Here's the drawing with two shaded views (mm, measured from the low corner). I have some questions. Round coordinates to 2 decimals unless told otherwise and drop trailing zeros. Write each loop counter-clockwise with the first axis right and the second up, starting at its lowest first coordinate (ties: lowest second). Pieces come first, ordered by that corner, then holes. Notation, with made-up numbers: M 52,-0.75 L 95,-0.75 A27 cw 95,24.25 Z; hole C 81.25,54.5 d1. An arc over 180 degrees is marked long. Use one line per item in the form item = value. Start each with the question number.
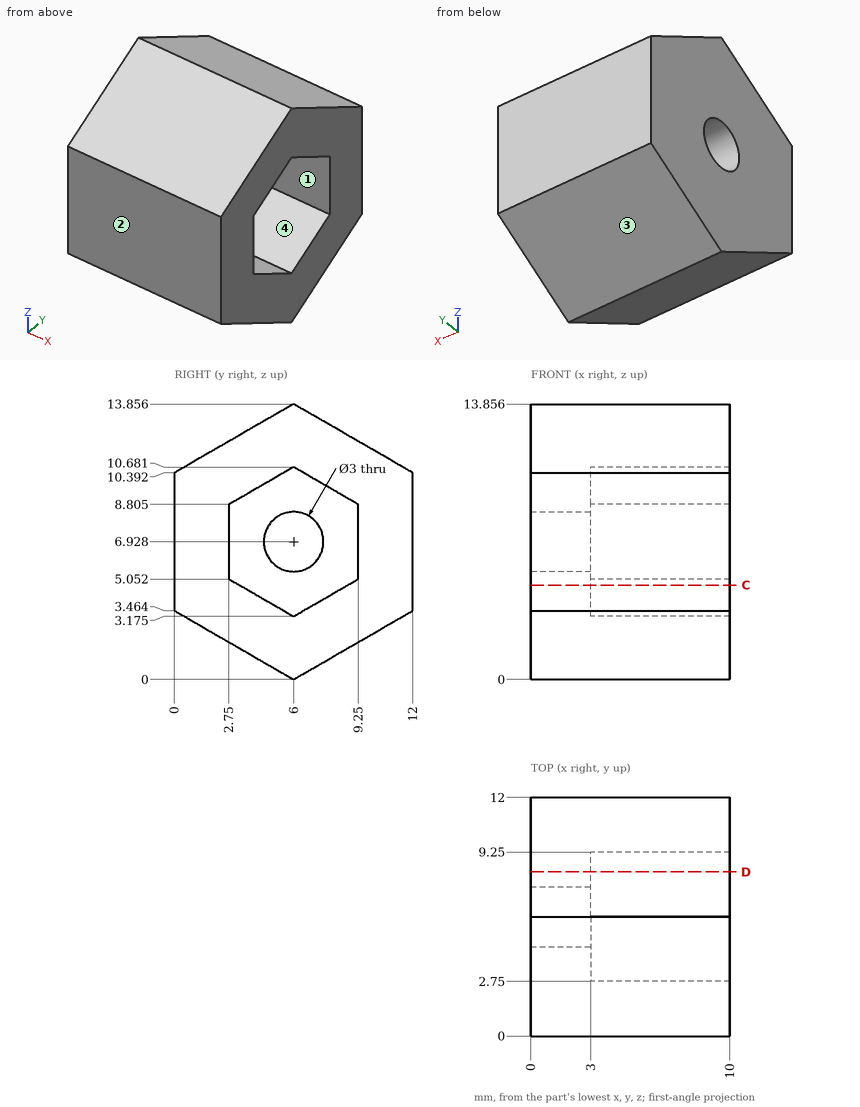
1. If we mould it in two halves opening along Y, with no side actions, what happens to the marked faces 1, 2, 3 and 4? For each: pulls with the +Y half, pulls with the -Y half, needs draft (parallel to the pull), parting line crosses it, or undercut.
2. Will these pins go through, and if not, where does the flat tip stop? pin 1 (4 mm diameter, centred on x = 3, y = 10, fed in from -Z) (1 decimal); pin 2 (2.5 mm diameter, centred on y = 6, z = 6.93, fed in from +X); pin 3 (6 mm diameter, centred on x = 3, y = 10, fed in from +Z).
3. If we section it at D-D (y = 8.25): List the corners of the cut face in (x, z) for me (1 decimal).
4. If we section it at C-C (z = 4.75): List the corners of the cut face in (x, y) for me.
5. Please list where these lines run through material, in increasing order: line 1 along Y through (x, z) = (7.25, 6.25); line 2 along X through (y, z) = (4.5, 8); line 3 along Y through (x, z) = (4.5, 9) (1 decimal).
Model answer:
q1.face_1 = undercut
q1.face_2 = pulls with the -Y half
q1.face_3 = pulls with the +Y half
q1.face_4 = undercut
q2.pin_1 = 1.2
q2.pin_2 = through
q2.pin_3 = 13.28
q3.outline = M 0,1.3 L 10,1.3 L 10,4.5 L 3,4.5 L 3,9.4 L 10,9.4 L 10,12.6 L 0,12.6 Z
q4.outline = M 0,0 L 10,0 L 10,3.27 L 3,3.27 L 3,8.73 L 10,8.73 L 10,12 L 0,12 Z
q5.line_1 = 0 to 2.75, 9.25 to 12
q5.line_2 = 0 to 3
q5.line_3 = 0 to 3.1, 8.9 to 12
